```python
from build123d import *

# Parameters (mm, degrees)
F0_R     = 16
F1_DEPTH = 55
F2_R     = 22
F3_DEPTH = 5
F5_D     = 28.4


with BuildPart() as f1:
    # F0 (on Top) → F1 (new body)
    with BuildSketch(Plane.XY):
        Circle(F0_R)
    extrude(amount=F1_DEPTH)

    # F2 (on Top) → F3 (join)
    with BuildSketch(Plane.XY):
        Circle(F2_R)
    extrude(amount=F3_DEPTH)

    # F5 (through all)
    with Locations(Plane(origin=(0, 0, 0), x_dir=(1, 0, 0), z_dir=(0, 0, -1))):
        with Locations((0, 0)):
            Hole(F5_D / 2)


solid = f1.part
```
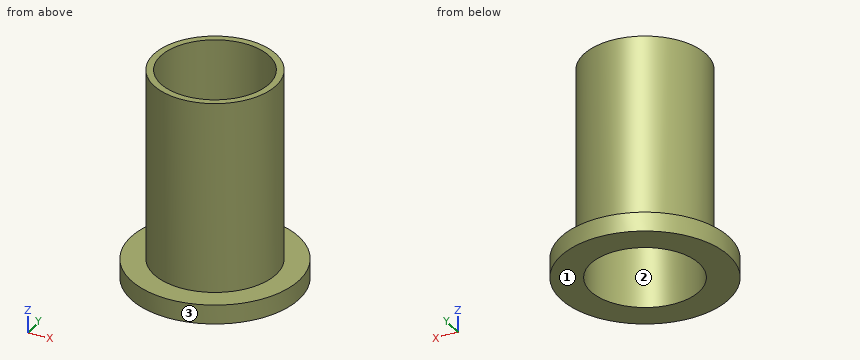
Design review of the part built by this model. Coordinates are the model's own, in mm. Face numbers are marked on the shaded views. Round coordinates to 2 decimals unless told otherwise and drop trailing zeros. Order: outer loops, then holes, each group sorted by start corner. A loop starts at its lowest first (then second) coordinate and runs counter-clockwise, first axis right, second up. Notation, with made-up numbers: (4.25, -38.5) - (54.25, -38.5) arc R25 cw to (54.25, -13.5) - close; hole circle Ø10 at (80.5, 67.25). An arc over 180 degrees is marked (long way). Return JSON: item names as keys, results as strings.
Q1. Consider section D-D on x = 19. Write out the cut boundary in (y, z), plus the area to 3 significant figures.
Computed values:
{"outline": "(-11.09, 0) - (11.09, 0) - (11.09, 5) - (-11.09, 5) - close", "area": "111 mm2"}
Q2. Consider section C-C on z = 43. Write out the cut boundary in (x, y).
Computed values:
{"outline": "circle Ø32 at (0, 0); hole circle Ø28.4 at (0, 0)"}
Q3. The part is to be moulded in two halves that separate along Y. For the marked faces 1, 2 and 3, say which applies: pulls with the +Y half, pulls with the -Y half, needs draft (parallel to the pull), parting line crosses it, or undercut.
Computed values:
{"face 1": "needs draft", "face 2": "undercut", "face 3": "parting line crosses it"}
Q4. Wall thickness on L1, parallel to Y at x = 0, z = 44; L2, parallel to Z at x = 20, y = 7.5; L3, parallel to Y at x = 12.5, z = 5.5: over which ranges is each line inside the solid? List them lowest first. Write a range as [from, to].
Computed values:
{"L1": "y = [-16, -14.2], [14.2, 16]", "L2": "z = [0, 5]", "L3": "y = [-9.99, -6.74], [6.74, 9.99]"}
Q5. Consider section A-A on x = 0. Write out the cut boundary in (y, z), plus the area to 3 significant figures.
Computed values:
{"outline": "(-22, 0) - (-14.2, 0) - (-14.2, 55) - (-16, 55) - (-16, 5) - (-22, 5) - close; (14.2, 0) - (22, 0) - (22, 5) - (16, 5) - (16, 55) - (14.2, 55) - close", "area": "258 mm2"}
Q6. For pin 1 Ø4 at (y, z) = (-3.5, 35) entering from +X; pin 2 Ø10 at (x, z) = (5, 17.5) entering from +Y; pin 3 Ø6 at (y, z) = (14, 32) entering from +X; pin 4 Ø8 at (x, y) = (7.5, -6) entering from +Z, all flat-tipped, find the tip position at first contact; note any pin that passes through.
Computed values:
{"pin 1": "stops at x = 15.93", "pin 2": "stops at y = 16", "pin 3": "stops at x = 11.62", "pin 4": "passes through"}
